Read the model definition and answer for the solid it produces. Units are mm, in the model's axes. Give positions to 0.01 mm unless a question says otherwise; leave off trailing zeros. Write each loop counter-clockwise with the first axis right and the second up, starting at its lowest first coordinate (ties: lowest second). Pieces come first, ordered by that corner, then holes. Notation, with made-up numbers: (-39, 7.5) -> (-23, 7.5) arc R17 cw to (-23, 40.5) -> close; hole circle Ø10 at (83.25, 45.5). An arc over 180 degrees is marked (long way). Write item = value, one per line.
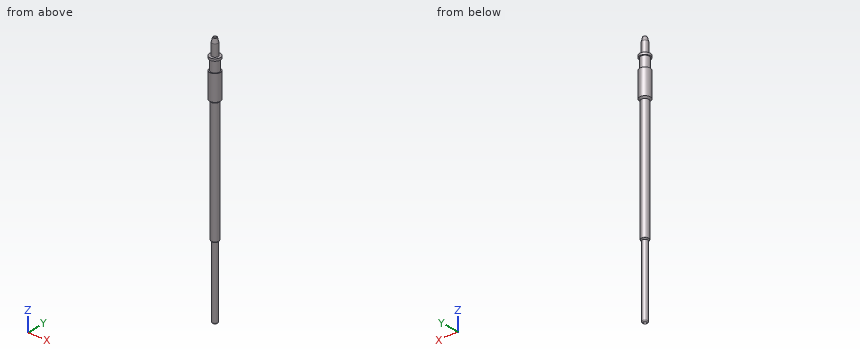
from build123d import *

# Parameters (mm, degrees)
F3_R        = 1.5
F4_DEPTH    = 235.059312583
F5_S5_R     = 3.5
F5_T6_DEPTH = 9
F6_SIZE2    = 4
F6_SIZE     = 1
F7_R        = 0.2
F8_R        = 0.5
F9_R        = 0.99999


# Not quite as in the source:
# - a fillet or chamfer that OpenCascade refuses, or shapes differently, is made with other operations: its cross-section is extruded or revolved along the edge and cut away or added
# - a fillet or chamfer is up to 0.001 mm smaller than in the source, because OpenCascade refuses the exact size


with BuildPart() as f1:
    # F0 (on Front) → F1 (revolve)
    with BuildSketch(Plane.XZ):
        Polygon((-1.5, -204.558312583), (-1.5, 29.441687417), (-2.75, 28.441687417), (-2.75, 14.441687417), (-5, 14.441687417), (-5, 12.441687417), (-4, 12.441687417), (-4, 2.241687417), (-5, 2.241687417), (-5, -22.258312583), (-3.5, -23.258312583), (-3.5, -136.558312583), (-2.5, -137.558312583), (-2.5, -204.558312583), align=None)
        Polygon((-5, -23.258312583), (-3.5, -23.258312583), (-5, -22.258312583), align=None)
        Polygon((-2.75, 28.441687417), (-1.5, 29.441687417), (-2.75, 29.441687417), align=None)
    revolve(axis=Axis((0, 0, -86.958312583), (0, 0, -1)))

    # F3 (on offset) → F4 (cut, through all)
    with BuildSketch(Plane.XY.offset(30.5)):
        Circle(F3_R)
    extrude(amount=-F4_DEPTH, mode=Mode.SUBTRACT)

    # F5: chamfer of 2 on 1 edges, made by hand


with BuildPart() as f5_tool2:
    # F5_s3 → F5_t4 (revolve)
    with BuildSketch(Plane.XZ):
        Polygon((-5, -21.258312583), (-3, -23.258312583), (-5, -23.258312583), align=None)
    revolve(axis=Axis((0, 0, -23.258312583), (0, 0, -1)))

    # F5_s5 → F5_t6 (cut, symmetric)
    with BuildSketch(Plane.XY.offset(-22.3)):
        Circle(F5_S5_R)
    extrude(amount=F5_T6_DEPTH, both=True, mode=Mode.SUBTRACT)


with BuildPart() as f1_1:
    add(f1.part)

    # F5_t1: cut F5_tool2
    add(f5_tool2.part, mode=Mode.SUBTRACT)

    # F6
    f6_edges = [f1_1.edges().sort_by_distance(p)[0] for p in [
        (2.75, 0, 29.441687),
    ]]
    chamfer(f6_edges, length=F6_SIZE, length2=F6_SIZE2)

    # F7
    f7_edges = [f1_1.edges().sort_by_distance(p)[0] for p in [
        (1.75, 0, 29.441687),
    ]]
    fillet(f7_edges, radius=F7_R)

    # F8
    f8_edges = [f1_1.edges().sort_by_distance(p)[0] for p in [
        (3.5, 0, -136.558313),
    ]]
    fillet(f8_edges, radius=F8_R)

    # F9 (radius 1 in the source; OpenCascade refuses exactly that, so slightly less here)
    f9_edges = [f1_1.edges().sort_by_distance(p)[0] for p in [
        (2.5, 0, -204.558313),
    ]]
    fillet(f9_edges, radius=F9_R)


solid = f1_1.part
(1) Consider L1, parallel to X at y = 0, z = -115; L2, parallel to X at y = -0.75, z = -133.5. Determine where each line is inside the solid, lowest interval first.
Checks:
L1 = -3.5 to -1.5, 1.5 to 3.5
L2 = -3.42 to -1.3, 1.3 to 3.42
(2) The part is cut by section B-B on z = -86. Determine the outline of the cut face in (x, y), plus the area to 3 significant figures.
Checks:
outline = circle Ø7 at (0, 0); hole circle Ø3 at (0, 0)
area = 31.4 mm²
(3) The part is cut by section A-A on z = -181. Determine the outline of the cut face in (x, y), plus the area to 3 significant figures.
Checks:
outline = circle Ø5 at (0, 0); hole circle Ø3 at (0, 0)
area = 12.6 mm²
(4) Given P1, Ø1, axis at x = -3, y = 4, coming from the -Z side; P2, Ø5, axis at x = 0, y = 0, coming from the +Z side; P3, Ø3, axis at x = -2.5, z = -147, coming from the +Y side; P4, Ø3, axis at y = 3.5, z = -131.5, coming from the -X side, each flat-ended and moving along its own axis, determine where each tip first touches the part or whether it passes through.
Checks:
P1 = -21.76
P2 = 29.44
P3 = 2.29
P4 = -2.87
